from build123d import *

# Parameters (mm, degrees)
F2_DEPTH  = 56.49083
F3_DEPTH  = 50.29662
F4_W      = 17.6400020719
F4_H      = 34.6500007436
F5_DEPTH  = 152.4
F6_W      = 8.1899985671
F6_H      = 40.634999983
F7_DEPTH  = 152.4
F8_R      = 1.7367288427
F9_W      = 11.1553873867
F9_H      = 10.141255334
F10_DEPTH = 26.2403


with BuildPart() as f2:
    # F0 (on Right) → F2 (new body, symmetric)
    with BuildSketch(Plane.YZ):
        Polygon((76.3685554266, 0), (-76.3685554266, 0), (-50.4032447934, -76.1139914393), (76.3685554266, -76.1139914393), align=None)
    extrude(amount=F2_DEPTH, both=True)

    # F1 (on face) → F3 (cut, symmetric)
    with BuildSketch(Plane.YZ):
        Polygon((69.2408159375, 0), (-67.0627951622, 0), (-43.7846407294, -68.349853158), (69.2408159375, -68.349853158), align=None)
    extrude(amount=F3_DEPTH, both=True, mode=Mode.SUBTRACT)

    # F4 (on Right) → F5 (cut, symmetric)
    with BuildSketch(Plane.YZ):
        with Locations((-75.7574997842, -6.6150003113)):
            Rectangle(F4_W, F4_H)
    extrude(amount=F5_DEPTH, both=True, mode=Mode.SUBTRACT)

    # F6 (on Right) → F7 (cut, symmetric)
    with BuildSketch(Plane.YZ):
        with Locations((-68.42822209, -15.2774997987)):
            Rectangle(F6_W, F6_H)
    extrude(amount=F7_DEPTH, both=True, mode=Mode.SUBTRACT)

    # F8
    f8_edges = [f2.edges().sort_by_distance(p)[0] for p in [
        (0, -64.333223, -8.014633),
    ]]
    fillet(f8_edges, radius=F8_R)

    # F9 (on face) → F10 (cut)
    with BuildSketch(Plane(origin=(0, 76.3685554266, 0), x_dir=(-1, 0, 0), z_dir=(0, 1, 0))):
        Polygon((-5.5776936933, -31.7187085748), (-13.1836356595, -31.7187085748), (-13.1836356595, -44.3952828646), (13.1836356595, -44.3952828646), (13.1836356595, -31.7187085748), (5.5776936933, -31.7187085748), (5.5776936933, -41.8599639088), (-5.5776936933, -41.8599639088), align=None)
        with Locations((0, -26.6480809078)):
            Rectangle(F9_W, F9_H)
        with Locations((0, -36.7893362418)):
            Rectangle(F9_W, F9_H)
    extrude(amount=-F10_DEPTH, mode=Mode.SUBTRACT)


solid = f2.part
Can you work these out from the model? Positions are in its coordinate system, mm. A direction names the side the tool comes from. Give positions to 0.01 mm unless a question says otherwise; leave off trailing zeros. Loops run counter-clockwise (first coordinate to the right, second up) from the corner with the lowest first, then second, coordinate; pieces in that order, holes last. Notation, with made-up numbers: (6.25, 13.25) - (11.25, 13.25) arc R21 ccw to (11.25, 21.25) - close; hole circle Ø11 at (51, 66.5). An arc over 180 degrees is marked (long way). Return JSON: item names as keys, results as strings.
1. We'd pull the mould along Z, two halves only. Please class faces 4 (the face through (5.578, 73, -27)), 5 (the face through (0.791, -57.466, -55.411)), 6 (the face through (-5.578, 73, -27)), 7 (the face through (-56.491, 5, -38)): +Z half, -Z half, draft (parallel to the pull), parting line (faces both ways), or undercut.
Output values:
{"face 4": "undercut", "face 5": "-Z half", "face 6": "undercut", "face 7": "draft"}
2. I want a section at D-D on x = 10. Please give me the cut outline in (y, z), and give its area (3 significant figures).
Output values:
{"outline": "(-64.33, -35.28) - (-50.4, -76.11) - (76.37, -76.11) - (76.37, -44.4) - (69.24, -44.4) - (69.24, -68.35) - (-43.78, -68.35) - (-60.95, -17.94) arc R1.74 ccw to (-64.33, -18.5) - close; (69.24, -31.72) - (76.37, -31.72) - (76.37, 0) - (69.24, 0) - close", "area": "1,810 mm²"}
3. I'm going to push flat-ended pins straight in: pin 1 Ø1 at (x, z) = (6, -36.5) entering from +Y; pin 2 Ø5 at (x, y) = (39.5, -3) entering from +Z; pin 3 Ø8 at (x, z) = (-39, -18) entering from -Y. Where does each tip first touch, or does it pass through?
Output values:
{"pin 1": "stops at y = -54.46", "pin 2": "stops at z = -68.35", "pin 3": "stops at y = -64.33"}
4. I want a section at B-B on z = -50.5. Please give me the cut outline in (x, y).
Output values:
{"outline": "(-56.49, -59.14) - (56.49, -59.14) - (56.49, 76.37) - (-56.49, 76.37) - close; hole (-50.3, -49.86) - (50.3, -49.86) - (50.3, 69.24) - (-50.3, 69.24) - close"}
5. If I drill on line 1 (X direction, y = 45, z = -6); line 2 (Z direction, x = 29, y = -32); line 3 (Y direction, x = 31.5, z = -6), over which ranges is the centre line in solid material (lowest first)?
Output values:
{"line 1": "x = -56.49 to -50.3, 50.3 to 56.49", "line 2": "z = -76.11 to -68.35", "line 3": "y = 69.24 to 76.37"}
6. For faces 1 (the face through (0.7, -52.49, -42.79)), 2 (the face through (-9, 73, -31.719)), 3 (the face through (1, 12, -76.114)), which set-ups out of +Z, -Z, +X, -X, +Y, -Y let a thin tool reach every point of the face, with its end or its side?
Output values:
{"face 1": "+Z", "face 2": "+Y", "face 3": "-Z, +X, -X, +Y, -Y"}
7. I want a section at C-C on y = 56. Please give me the cut outline in (x, z).
Output values:
{"outline": "(-56.49, -76.11) - (56.49, -76.11) - (56.49, 0) - (50.3, 0) - (50.3, -68.35) - (-50.3, -68.35) - (-50.3, 0) - (-56.49, 0) - close"}
8. I want a section at A-A on x = -1.5. Please give me the cut outline in (y, z).
Output values:
{"outline": "(-64.33, -35.28) - (-50.4, -76.11) - (76.37, -76.11) - (76.37, -44.4) - (69.24, -44.4) - (69.24, -68.35) - (-43.78, -68.35) - (-60.95, -17.94) arc R1.74 ccw to (-64.33, -18.5) - close; (69.24, -21.58) - (76.37, -21.58) - (76.37, 0) - (69.24, 0) - close"}
